Work out the finished part from the listing and answer in its coordinate system (mm). A direction names the side the tool comes from. Coordinates: 2 decimals unless noted, no trailing zeros. Write each loop counter-clockwise with the first axis right and the second up, starting at its lowest first coordinate (ties: lowest second). Pieces come first, ordered by that corner, then holes. Notation, with made-up numbers: (10, 81.25) - (21, 81.25) arc R11 ccw to (21, 101.25) - close; hole circle Ø8 at (72, 40). An arc over 180 degrees is marked (long way). Use one line per item in the form item = value. Start each with the question number.
Item 1: A cutting plane is placed at C-C (z = 13). Write down the section's boundary in (x, y).
Item 2: A cutting plane is placed at A-A (y = -184). Write down the section's boundary in (x, z).
Item 3: A cutting plane is placed at D-D (y = 55.5). Write down the section's boundary in (x, z), then the cut area to 3 significant figures.
Item 4: Given pin 1 (8.5 mm diameter, centred on x = 44, z = 240, fed in from -Y); pin 2 (23 mm diameter, centred on y = 55, z = 77.5, fed in from +X); pin 3 (3 mm diameter, centred on x = -95, z = 187.5, fed in from -Y), each flat-ended and moving along its own axis, determine where each tip first touches the part or whether it passes through.
Item 5: For faces 1 (the flat face through (15, 0, 88)), 2 (the flat face through (-184.162, -4, 83)), 3 (the flat face through (47, 59, -66.968)), determine the directions among +Z, -Z, +X, -X, +Y, -Y from which every point of the face is accessible in a straight line to the end or side of a thin tool.
Item 6: Consider probe 1 along Y at (x, z) = (116, 161.5); probe 2 along Z at (x, y) = (171, 97); probe 3 along Y at (x, z) = (-146.5, 131). Determine where each line is inside the solid, lowest interval first.
Item 7: Determine the mould class of faces 4 (the flat face through (15, -12, -66.968)), 5 (the flat face through (47, 97.784, 83)), 6 (the flat face through (12, 53, -79.668)), 7 (the flat face through (158, -254, 244)) for opening direction Z: released by +Z, released by -Z, zero draft, split by the parting line, or undercut.
Item 8: A cutting plane is placed at B-B (x = -98.5). Write down the section's boundary in (y, z).
from build123d import *

# Parameters (mm, degrees)
F1_DEPTH = 25.4
F2_W     = 76.2
F2_H     = 12.7
F3_DEPTH = 228.6
F4_W     = 368.3
F4_H     = 304.8
F5_DEPTH = 254
F6_R     = 5.08
F7_W     = 76.2
F7_H     = 304.8
F8_DEPTH = 304.8


with BuildPart() as f1:
    # F0 (on Front) → F1 (new body)
    with BuildSketch(Plane.XZ):
        Polygon((-171.4616481543, -66.9675160527), (-171.4616481543, 237.8324839473), (196.8383518457, 237.8324839473), (196.8383518457, 250.5324839473), (-184.1616481543, 250.5324839473), (-184.1616481543, -79.6675160527), (196.8383518457, -79.6675160527), (196.8383518457, -66.9675160527), align=None)
    extrude(amount=F1_DEPTH)

    # F2 (on face) → F3 (join)
    with BuildSketch(Plane.XZ.offset(25.4)):
        Polygon((-82.5616481543, 237.8324839473), (-82.5616481543, 250.5324839473), (-184.1616481543, 250.5324839473), (-184.1616481543, -79.6675160527), (-82.5616481543, -79.6675160527), (-82.5616481543, -66.9675160527), (-171.4616481543, -66.9675160527), (-171.4616481543, 237.8324839473), align=None)
        with Locations((158.7383518457, 244.1824839473)):
            Rectangle(F2_W, F2_H)
        with Locations((158.7383518457, -73.3175160527)):
            Rectangle(F2_W, F2_H)
    extrude(amount=F3_DEPTH)

    # F4 (on face) → F5 (join)
    with BuildSketch(Plane(origin=(0, 0, 0), x_dir=(-1, 0, 0), z_dir=(0, 1, 0))):
        with Locations((-12.6883518457, 85.4324839473)):
            Rectangle(F4_W, F4_H)
        Polygon((184.1616481543, 250.5324839473), (-196.8383518457, 250.5324839473), (-196.8383518457, 237.8324839473), (171.4616481543, 237.8324839473), (171.4616481543, -66.9675160527), (-196.8383518457, -66.9675160527), (-196.8383518457, -79.6675160527), (184.1616481543, -79.6675160527), align=None)
    extrude(amount=F5_DEPTH)

    # F6
    f6_edges = [f1.edges().sort_by_distance(p)[0] for p in [
        (-184.161648, 0, -79.667516),
        (-184.161648, 0, 250.532484),
        (-82.561648, -139.7, -79.667516),
        (120.638352, -139.7, -79.667516),
        (19.038352, -25.4, -79.667516),
        (120.638352, -139.7, 250.532484),
        (19.038352, -25.4, 250.532484),
        (-82.561648, -139.7, 250.532484),
    ]]
    fillet(f6_edges, radius=F6_R)

    # F7 (on face) → F8 (cut)
    with BuildSketch(Plane.YZ.offset(196.8383518457)):
        with Locations((59.6839594603, 85.4324839473)):
            Rectangle(F7_W, F7_H)
    extrude(amount=-F8_DEPTH, mode=Mode.SUBTRACT)


solid = f1.part
Answer:
q1.outline = (-184.16, -254) - (-171.46, -254) - (-171.46, 0) - (196.84, 0) - (196.84, 21.58) - (-107.96, 21.58) - (-107.96, 97.78) - (196.84, 97.78) - (196.84, 254) - (-184.16, 254) - close
q2.outline = (-184.16, -74.59) arc R5.08 ccw to (-179.08, -79.67) - (-87.64, -79.67) arc R5.08 ccw to (-82.56, -74.59) - (-82.56, -66.97) - (-171.46, -66.97) - (-171.46, 237.83) - (-82.56, 237.83) - (-82.56, 245.45) arc R5.08 ccw to (-87.64, 250.53) - (-179.08, 250.53) arc R5.08 ccw to (-184.16, 245.45) - close; (120.64, -74.59) arc R5.08 ccw to (125.72, -79.67) - (196.84, -79.67) - (196.84, -66.97) - (120.64, -66.97) - close; (120.64, 237.83) - (196.84, 237.83) - (196.84, 250.53) - (125.72, 250.53) arc R5.08 ccw to (120.64, 245.45) - close
q3.outline = (-184.16, -74.59) arc R5.08 ccw to (-179.08, -79.67) - (196.84, -79.67) - (196.84, -66.97) - (-107.96, -66.97) - (-107.96, 237.83) - (196.84, 237.83) - (196.84, 250.53) - (-179.08, 250.53) arc R5.08 ccw to (-184.16, 245.45) - close
q3.area = 32,900 mm²
q4.pin_1 = -25.4
q4.pin_2 = -107.96
q4.pin_3 = 0
q5.face_1 = +X, -Y
q5.face_2 = +Z, -Z, -X, +Y, -Y
q5.face_3 = +X
q6.probe_1 = 0 to 21.58, 97.78 to 254
q6.probe_2 = -79.67 to -66.97, 237.83 to 250.53
q6.probe_3 = 0 to 254
q7.face_4 = undercut
q7.face_5 = undercut
q7.face_6 = released by -Z
q7.face_7 = zero draft
q8.outline = (-254, -79.67) - (254, -79.67) - (254, 250.53) - (-254, 250.53) - (-254, 237.83) - (0, 237.83) - (0, -66.97) - (-254, -66.97) - close; hole (21.58, -66.97) - (97.78, -66.97) - (97.78, 237.83) - (21.58, 237.83) - close
